```python
from build123d import *

# Parameters (mm, degrees)
SKETCH_R      = 2
PAD_DEPTH     = 6
SKETCH001_W   = 3
SKETCH001_H   = 20
SKETCH001_W_2 = 20
SKETCH001_H_2 = 3
PAD001_DEPTH  = 15
POCKET_DEPTH  = 4


with BuildPart() as part:
    # Sketch → Pad (new body)
    with BuildSketch(Plane.XY):
        with BuildLine():
            Line((-7, 12), (25, 12))
            Line((25, 12), (25, 15))
            Line((25, 15), (45, 15))
            Line((45, 15), (45, 0))
            Line((0, -45), (45, 0))
            Line((-15, -45), (0, -45))
            Line((-15, -25), (-15, -45))
            Line((-12, -25), (-15, -25))
            Line((-12, 7), (-12, -25))
            ThreePointArc((-7, 12), (-10.535534, 10.535534), (-12, 7))
        make_face()
        with Locations((31.564971, -7.778175)):
            Circle(SKETCH_R, mode=Mode.SUBTRACT)
        with Locations((7.778175, -31.564971)):
            Circle(SKETCH_R, mode=Mode.SUBTRACT)
    extrude(amount=PAD_DEPTH)

    # Sketch001 → Pad001 (join)
    with BuildSketch(Plane.XY):
        with Locations((-13.5, -35)):
            Rectangle(SKETCH001_W, SKETCH001_H)
        with Locations((35, 13.5)):
            Rectangle(SKETCH001_W_2, SKETCH001_H_2)
    extrude(amount=PAD001_DEPTH)

    # Sketch002 (on DatumPlane) → Pocket (cut)
    with BuildSketch(Plane.XY.offset(6)):
        Polygon((45, 0), (30, 0), (0, -30), (0, -45), align=None)
    extrude(amount=-POCKET_DEPTH, mode=Mode.SUBTRACT)


solid = part.part
```
The model under review builds one solid part; all positions refer to its coordinate system, in mm. A direction names the side the tool comes from. Round coordinates to 2 decimals unless told otherwise and drop trailing zeros. Write each loop counter-clockwise with the first axis right and the second up, starting at its lowest first coordinate (ties: lowest second). Pieces come first, ordered by that corner, then holes. Notation, with made-up numbers: (-32.75, -16) - (-4.75, -16) arc R19 ccw to (-4.75, -12) - close; hole circle Ø3 at (65, -29.75). An arc over 180 degrees is marked (long way). One line per question, with ' | ' between items.
Item 1: Add section B-B, the plane y = -38.5. Give the boundary of the cut face in (x, z).
Resolved:
outline: (-15, 0) - (6.5, 0) - (6.5, 2) - (0, 2) - (0, 6) - (-12, 6) - (-12, 15) - (-15, 15) - close
Item 2: Add section C-C, the plane x = 34.5. Give the boundary of the cut face in (y, z).
Resolved:
outline: (-10.5, 0) - (15, 0) - (15, 15) - (12, 15) - (12, 6) - (0, 6) - (0, 2) - (-10.5, 2) - close
Item 3: Add section D-D, the plane z = 5.25. Give the boundary of the cut face in (x, y).
Resolved:
outline: (-15, -45) - (0, -45) - (0, -30) - (30, 0) - (45, 0) - (45, 15) - (25, 15) - (25, 12) - (-7, 12) arc R5 ccw to (-12, 7) - (-12, -25) - (-15, -25) - close
Item 4: For P1, Ø22.5, axis at x = 21, y = -28, coming from the +Z side; P2, Ø8, axis at x = 24.5, y = -0.5, coming from the +Z side; P3, Ø0.9, axis at x = -13.5, z = 4.5, coming from the +Y side; P4, Ø5, axis at x = 31.56, y = -7.78, coming from the -Z side, all flat-tipped, find the tip position at first contact; note any pin that passes through.
Resolved:
P1: stops at z = 2 | P2: stops at z = 6 | P3: stops at y = -25 | P4: stops at z = 0
Item 5: The part is to be moulded in two halves that separate along Y. For faces 1 (the face through (33.412, -8.544, 0.986)), 2 (the face through (35, 12, 10)), 3 (the face through (45, 9, 4)), say which applies: pulls with the +Y half, pulls with the -Y half, needs draft (parallel to the pull), parting line crosses it, or undercut.
Resolved:
face 1: undercut | face 2: pulls with the -Y half | face 3: needs draft
Item 6: To check wall thickness, follow probe 1 along Z at (x, y) = (23, 7); probe 2 along X at (y, z) = (-29, 13); probe 3 along Y at (x, z) = (36, 2.5). State the ranges of each line that lie inside material, in increasing order.
Resolved:
probe 1: z = 0 to 6 | probe 2: x = -15 to -12 | probe 3: y = 0 to 15
Item 7: Add section A-A, the plane z = 13.5. Give the boundary of the cut face in (x, y), then the cut area to 3 significant figures.
Resolved:
outline: (-15, -45) - (-12, -45) - (-12, -25) - (-15, -25) - close; (25, 12) - (45, 12) - (45, 15) - (25, 15) - close | area: 120 mm2
Item 8: For faces 4 (the face through (15, -15, 4)), 5 (the face through (9, 12, 3)), 6 (the face through (7.345, -33.517, 0.986)), list the 3-axis set-ups (+Z, -Z, +X, -X, +Y, -Y) from which the entire face can be reached by the end or side of a thin tool; tool diameter is ignored.
Resolved:
face 4: +Z, +X, -Y | face 5: +Z, -Z, -X, +Y | face 6: +Z, -Z
